```python
from build123d import *

# Parameters (mm, degrees)
EXTRUDE_1_DEPTH     = 26
SKETCH_2_R          = 4.25
CUT_EXTRUDE_1_DEPTH = 5
SKETCH_3_R          = 4.25
CUT_EXTRUDE_2_DEPTH = 5
FILLET_1_R          = 4
FILLET_2_R          = 1


with BuildPart() as part:
    # Эскиз1 → Бобышка-Вытянуть1 (new body, symmetric)
    with BuildSketch(Plane.XY):
        Polygon((0, 0), (42.426406871, 42.426406871), (45.961940777, 38.890872965), (22.85244978, 15.781381968), (27.318244413, 5), (60, 5), (60, 0), align=None)
        Polygon((20.556349186, 13.485281374), (24.071067812, 5), (12.071067812, 5), align=None, mode=Mode.SUBTRACT)
    extrude(amount=EXTRUDE_1_DEPTH, both=True)

    # Эскиз2 → Вырез-Вытянуть1 (cut)
    with BuildSketch(Plane(origin=(0, 0, 0), x_dir=(0, 0, 1), z_dir=(-0.707106781, 0.707106781, 0))):
        with Locations(Location((-15, 45, 0), (0, 0, 270))):  # turned: the seam where the file's is
            Circle(SKETCH_2_R)
        with Locations(Location((15, 45, 0), (0, 0, 270))):  # turned: the seam where the file's is
            Circle(SKETCH_2_R)
    extrude(amount=-CUT_EXTRUDE_1_DEPTH, mode=Mode.SUBTRACT)

    # Эскиз3 → Вырез-Вытянуть2 (cut)
    with BuildSketch(Plane.XZ):
        with Locations(Location((45, 15, 0), (0, 0, 270))):  # turned: the seam where the file's is
            Circle(SKETCH_3_R)
        with Locations(Location((45, -15, 0), (0, 0, 270))):  # turned: the seam where the file's is
            Circle(SKETCH_3_R)
    extrude(amount=-CUT_EXTRUDE_2_DEPTH, mode=Mode.SUBTRACT)

    # Скругление1
    fillet_1_edges = [part.edges().sort_by_distance(p)[0] for p in [
        (45.961940777, 38.890872965, 0),
        (60, 5, 0),
    ]]
    fillet(fillet_1_edges, radius=FILLET_1_R)

    # Скругление2
    fillet_2_edges = [part.edges().sort_by_distance(p)[0] for p in [
        (20.556349186, 13.485281374, 0),
        (12.071067812, 5, 0),
        (24.071067812, 5, 0),
    ]]
    fillet(fillet_2_edges, radius=FILLET_2_R)


solid = part.part
```
Verification items for the finished model (mm, model axes). A direction names the side the tool comes from. Coordinates: 2 decimals unless noted, no trailing zeros. Loops run counter-clockwise (first coordinate to the right, second up) from the corner with the lowest first, then second, coordinate; pieces in that order, holes last. Notation, with made-up numbers: (25, 81.25) -> (66, 81.25) arc R8 cw to (66, 85.25) -> close; hole circle Ø11 at (56.25, 26). An arc over 180 degrees is marked (long way). Put each result on its own line as item: value.
1. Section check A-A, the plane z = -8. Record the boundary of the cut face in (x, y), then the cut area to 3 significant figures.
Result set:
outline: (0, 0) -> (60, 0) -> (60, 1) arc R4 ccw to (56, 5) -> (27.32, 5) -> (22.85, 15.78) -> (43.13, 36.06) arc R4 ccw to (43.13, 41.72) -> (42.43, 42.43) -> close; hole (13.78, 6.71) arc R1 ccw to (14.49, 5) -> (22.57, 5) arc R1 ccw to (23.5, 6.38) -> (21.13, 12.1) arc R1 ccw to (19.5, 12.43) -> close
area: 566 mm^2
2. Tool access check on faces 1 (the face through (40.85, 2.46, -14.08)), 2 (the face through (41, 5, 0)), 3 (the face through (16.6, 9.53, 0.36)). Record the directions out of +Z, -Z, +X, -X, +Y, -Y that give a thin tool (end or side, any length) a straight path to the whole face; none if there is none.
Result set:
face 1: -Y
face 2: +Z, -Z, +X
face 3: +Z, -Z
3. Gauge pin test, flat ends, axial feed: P1, Ø1, axis at x = 28, z = 15, coming from the +Y side; P2, Ø4, axis at y = 32.5, z = -7, coming from the +X side; P3, Ø4, axis at y = 38, z = 5, coming from the +X side. Record the tip position at first contact, or that the pin passes through.
Result set:
P1: stops at y = 28.5
P2: stops at x = 41.57
P3: stops at x = 44.31
4. Thickness scan on line 1 (Y direction, x = 14.5, z = -1); line 2 (Y direction, x = 55, z = 1.5); line 3 (Y direction, x = 28.5, z = 3.5). Record the ranges inside material, lowest first.
Result set:
line 1: y = 0 to 5, 7.43 to 14.5
line 2: y = 0 to 5
line 3: y = 0 to 5, 21.43 to 28.5
5. Section check D-D, the plane y = 18.5. Record the boundary of the cut face in (x, z).
Result set:
outline: (18.5, -26) -> (25.57, -26) -> (25.57, 26) -> (18.5, 26) -> close
6. Section check C-C, the plane x = 17.5. Record the boundary of the cut face in (y, z).
Result set:
outline: (0, -26) -> (5, -26) -> (5, 26) -> (0, 26) -> close; (10.43, -26) -> (17.5, -26) -> (17.5, 26) -> (10.43, 26) -> close
7. Mould release check, pull along X, two halves, no side actions. Record for faces 4 (the face through (23, 12, -26)), 5 (the face through (23.413, 5.456, 0.364)), 6 (the face through (33.13, 26.06, 0.36)), 7 (the face through (21, 21, 0)): pulls with the +X half, pulls with the -X half, needs draft (parallel to the pull), parting line crosses it, or undercut.
Result set:
face 4: needs draft
face 5: undercut
face 6: pulls with the +X half
face 7: pulls with the -X half
8. Section check B-B, the plane z = -13.5. Record the boundary of the cut face in (x, y), then the cut area to 3 significant figures.
Result set:
outline: (0, 0) -> (41.02, 0) -> (41.02, 5) -> (27.32, 5) -> (22.85, 15.78) -> (32.54, 25.47) -> (29.01, 29.01) -> close; (34.63, 34.63) -> (38.17, 31.1) -> (43.13, 36.06) arc R4 ccw to (43.13, 41.72) -> (42.43, 42.43) -> close; (48.98, 0) -> (60, 0) -> (60, 1) arc R4 ccw to (56, 5) -> (48.98, 5) -> close; hole (13.78, 6.71) arc R1 ccw to (14.49, 5) -> (22.57, 5) arc R1 ccw to (23.5, 6.38) -> (21.13, 12.1) arc R1 ccw to (19.5, 12.43) -> close
area: 487 mm^2
